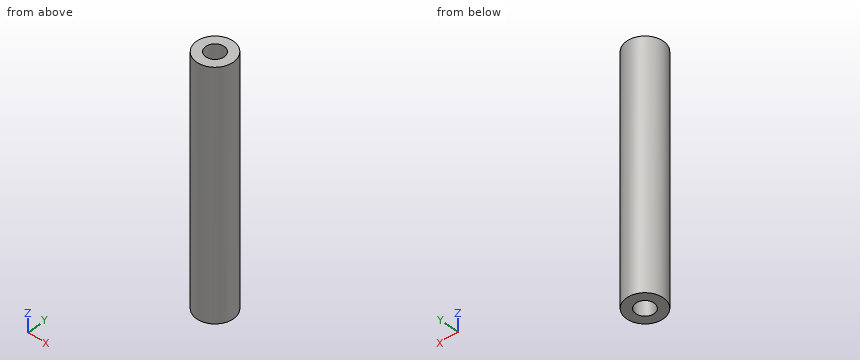
Autodesk Inventor part; units mm, degrees
ref_plane "YZ Plane" through (0, 0, 0) normal (1, 0, 0) x (0, 1, 0)
ref_plane "XZ Plane" through (0, 0, 0) normal (0, 1, 0) x (-1, 0, 0)
ref_plane "XY Plane" through (0, 0, 0) normal (0, 0, 1) x (1, 0, 0)
sketch "Sketch1" plane through (0, 0, 0) normal (0, 0, 1) x (1, 0, 0)
  circle A0 centre (0, 0) radius 1.25
  circle A1 centre (0, 0) radius 3
  dimension "d0" = 2.5
  dimension "d1" = 6
extrude "Extrusion1" add sketch "Sketch1" against normal blind 40 contours A0 | A1
sketch "スケッチ2" plane through (0, 0, 0) normal (0, 0, 1) x (1, 0, 0)
  circle A0 centre (0, 0) radius 1.5
  dimension "d4" = 3
extrude "押し出し2" cut sketch "スケッチ2" against normal blind 6
sketch "スケッチ3" plane through (0, 0, -40) normal (0, 0, -1) x (-1, 0, 0)
  circle A0 centre (0, 0) radius 1.5
extrude "押し出し3" cut sketch "スケッチ3" against normal blind 6
properties part number "l40" material "Aluminum 2014-T4"
Could you check a few things on this model? Use its own coordinates, in mm. Round coordinates to 2 decimals unless told otherwise and drop trailing zeros. Write each loop counter-clockwise with the first axis right and the second up, starting at its lowest first coordinate (ties: lowest second). Pieces come first, ordered by that corner, then holes. Notation, with made-up numbers: (53.5, 27) -> (61.5, 27) arc R35 ccw to (61.5, 61) -> close; hole circle Ø11 at (86, 59). An arc over 180 degrees is marked (long way). Use a Markdown table: item, result.
1. For pin 1 Ø3 at (x, z) = (2.5, -24.5) entering from +Y; pin 2 Ø1.5 at (x, z) = (0.5, -20) entering from -Y; pin 3 Ø1.5 at (x, y) = (-0.5, 0.5) entering from -Z; pin 4 Ø1.8 at (x, y) = (0, 0) entering from +Z, each with a flat end and sliding along its axis, tell me the tip position at first contact or that it passes through.
Answer key:
| item | result |
|---|---|
| pin 1 | stops at y = 2.83 |
| pin 2 | stops at y = -3 |
| pin 3 | stops at z = -34 |
| pin 4 | stops at z = -6 |
2. Please list where these lines run through material, in increasing order: probe 1 along Y at (x, z) = (0, -1.35); probe 2 along Z at (x, y) = (0.85, 0.1); probe 3 along Y at (x, z) = (1, -34.5).
Answer key:
| item | result |
|---|---|
| probe 1 | y = -3 to -1.5, 1.5 to 3 |
| probe 2 | z = -34 to -6 |
| probe 3 | y = -2.83 to -1.12, 1.12 to 2.83 |
3. If we section it at D-D (y = -2.4): List the corners of the cut face in (x, z) for me.
Answer key:
| item | result |
|---|---|
| outline | (-1.8, -40) -> (1.8, -40) -> (1.8, 0) -> (-1.8, 0) -> close |
4. If we section it at A-A (x = 0): List the corners of the cut face in (y, z) for me.
Answer key:
| item | result |
|---|---|
| outline | (-3, -40) -> (-1.5, -40) -> (-1.5, -34) -> (1.5, -34) -> (1.5, -40) -> (3, -40) -> (3, 0) -> (1.5, 0) -> (1.5, -6) -> (-1.5, -6) -> (-1.5, 0) -> (-3, 0) -> close |
5. If we section it at C-C (z = -17.5): List the corners of the cut face in (x, y) for me.
Answer key:
| item | result |
|---|---|
| outline | circle Ø6 at (0, 0) |
